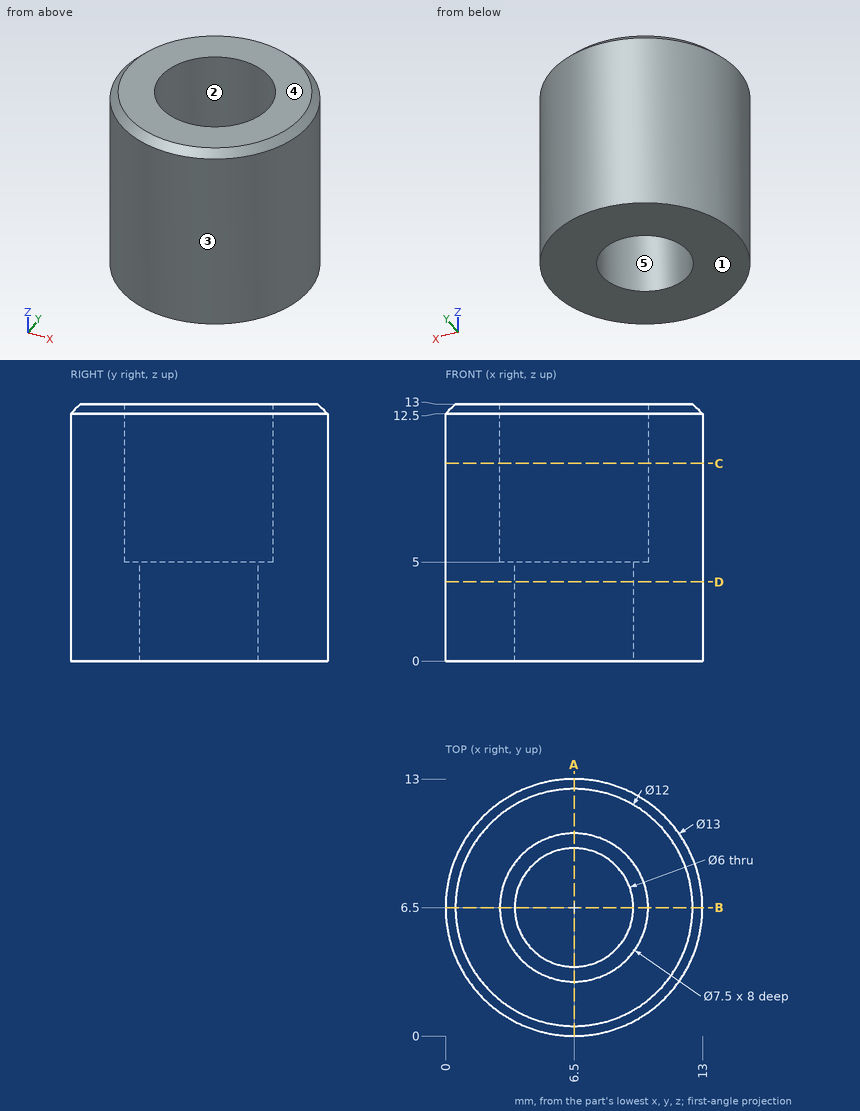
Part print with two shaded views. Sizes in mm from the minimum x, y, z corner. A direction names the side the tool comes from. Round coordinates to 2 decimals unless told otherwise and drop trailing zeros. Loops run counter-clockwise (first coordinate to the right, second up) from the corner with the lowest first, then second, coordinate; pieces in that order, holes last. Notation, with made-up numbers: (-26, 66.25) - (28, 66.25) arc R25 ccw to (28, 94.25) - close; hole circle Ø2 at (48.25, 54). An arc over 180 degrees is marked (long way). Put each result on its own line as item: value.
1. 3-axis set-ups, long thin cutter, end or side, ignore diameter. For the marked faces 1 and 2: which of +Z, -Z, +X, -X, +Y, -Y reach the whole face in a straight line?
Geometry check:
face 1: -Z, +X, -X, +Y, -Y
face 2: +Z
2. Pin check, flat tips, straight feed: P1, Ø2, axis at x = 7.5, y = 6.5, coming from the +Z side; P2, Ø6, axis at x = 9, z = 7, coming from the -Y side; P3, Ø1, axis at y = 3.5, z = 4.5, coming from the +X side; P4, Ø1, axis at y = 10.5, z = 7, coming from the -X side. Stop position of each tip, or through.
Geometry check:
P1: through
P2: y = 0
P3: x = 12.5
P4: x = 1.02
3. Two-plate mould, pull along Y, no slides. Class the marked faces 3, 4 and 5: released by +Y, released by -Y, zero draft, split by the parting line, or undercut.
Geometry check:
face 3: split by the parting line
face 4: zero draft
face 5: undercut
4. Slice it at D-D on z = 4. List the corners of the cut face in (x, y).
Geometry check:
outline: circle Ø13 at (6.5, 6.5); hole circle Ø6 at (6.5, 6.5)
5. Slice it at C-C on z = 10. List the corners of the cut face in (x, y), and give its area (3 significant figures).
Geometry check:
outline: circle Ø13 at (6.5, 6.5); hole circle Ø7.5 at (6.5, 6.5)
area: 88.6 mm²
6. Slice it at A-A on x = 6.5. List the corners of the cut face in (y, z), and give its area (4 significant figures).
Geometry check:
outline: (0, 0) - (3.5, 0) - (3.5, 5) - (2.75, 5) - (2.75, 13) - (0.5, 13) - (0, 12.5) - close; (9.5, 0) - (13, 0) - (13, 12.5) - (12.5, 13) - (10.25, 13) - (10.25, 5) - (9.5, 5) - close
area: 78.75 mm²
7. Wall check: line 1 (Y direction, x = 6.5, z = 11.25); line 2 (Z direction, x = 9.75, y = 6.75); line 3 (Y direction, x = 4, z = 2.5). Give the ranges that are in metal, low to high.
Geometry check:
line 1: 0 to 2.75, 10.25 to 13
line 2: 0 to 5
line 3: 0.5 to 4.84, 8.16 to 12.5
